```python
from build123d import *

# Parameters (mm, degrees)
SKETCH1_R           = 2.5
BOSS_EXTRUDE1_DEPTH = 6
CUT_EXTRUDE2_DEPTH  = 41.954878106


with BuildPart() as part:
    # Sketch1 → Boss-Extrude1 (new body)
    with BuildSketch(Plane.XY):
        with BuildLine():
            Line((3, 37.066220694), (3, 28.566220694))
            ThreePointArc((3, 28.566220694), (0, 25.566220694), (-3, 28.566220694))
            Line((-3, 28.566220694), (-3, 37.066220694))
            ThreePointArc((-3, 37.066220694), (0, 40.066220694), (3, 37.066220694))
        make_face()
        with Locations((0, 37.066220694)):
            Circle(SKETCH1_R, mode=Mode.SUBTRACT)
        with Locations((0, 28.566220694)):
            Circle(SKETCH1_R, mode=Mode.SUBTRACT)
    extrude(amount=BOSS_EXTRUDE1_DEPTH)

    # Sketch2 → Cut-Extrude2 (cut, through all)
    with BuildSketch(Plane.ZY.offset(3)):
        Polygon((2, 37.066220694), (2, 41.792397486), (4, 41.792397486), (4, 37.066220694), (4, 32.376323295), (2, 32.376323295), align=None)
    extrude(amount=-CUT_EXTRUDE2_DEPTH, mode=Mode.SUBTRACT)


solid = part.part
```
Geometry check sheet. Reference: the model listing, model coordinates, mm. A direction names the side the tool comes from. Round coordinates to 2 decimals unless told otherwise and drop trailing zeros. Loops run counter-clockwise (first coordinate to the right, second up) from the corner with the lowest first, then second, coordinate; pieces in that order, holes last. Notation, with made-up numbers: (36, 14.25) -> (72, 14.25) arc R17 cw to (72, 39.25) -> close; hole circle Ø5 at (57, 44). An arc over 180 degrees is marked (long way). Use a Markdown table: item, result.
(1) Mould release check, pull along Y, two halves, no side actions. Record for faces 1 (the cylindrical face through (0.066, 25.567, 2.958)), 2 (the flat face through (-1.4, 34.6, 2)), 3 (the cylindrical face through (-0.325, 31.045, 2.958)), 4 (the cylindrical face through (1.3, 39.2, 1)): released by +Y, released by -Y, zero draft, split by the parting line, or undercut.
Calculated:
| item | result |
|---|---|
| face 1 | released by -Y |
| face 2 | zero draft |
| face 3 | undercut |
| face 4 | undercut |
(2) Sectioned sample at A-A (x = 0). Enter the section's corners in (y, z), then the cut area to 3 significant figures.
Calculated:
| item | result |
|---|---|
| outline | (25.57, 0) -> (26.07, 0) -> (26.07, 6) -> (25.57, 6) -> close; (31.07, 0) -> (34.57, 0) -> (34.57, 2) -> (32.38, 2) -> (32.38, 4) -> (34.57, 4) -> (34.57, 6) -> (31.07, 6) -> close; (39.57, 0) -> (40.07, 0) -> (40.07, 2) -> (39.57, 2) -> close; (39.57, 4) -> (40.07, 4) -> (40.07, 6) -> (39.57, 6) -> close |
| area | 21.6 mm² |
(3) Sectioned sample at C-C (y = 36.25). Enter the section's corners in (x, z), then the cut area to 3 significant figures.
Calculated:
| item | result |
|---|---|
| outline | (-3, 0) -> (-2.36, 0) -> (-2.36, 2) -> (-3, 2) -> close; (-3, 4) -> (-2.36, 4) -> (-2.36, 6) -> (-3, 6) -> close; (2.36, 0) -> (3, 0) -> (3, 2) -> (2.36, 2) -> close; (2.36, 4) -> (3, 4) -> (3, 6) -> (2.36, 6) -> close |
| area | 5.10 mm² |
(4) Go/stop test with flat-tipped pins: P1, Ø1.5, axis at x = 1, z = 4.5, coming from the -Y side; P2, Ø3, axis at y = 37.5, z = 1, coming from the -X side; P3, Ø1, axis at x = -0.5, z = 3, coming from the +Y side. Record where each tip stops, or that it passes through.
Calculated:
| item | result |
|---|---|
| P1 | y = 25.58 |
| P2 | x = -3 |
| P3 | y = 32.38 |
(5) Sectioned sample at B-B (z = 4.65). Enter the section's corners in (x, y), then the cut area to 3 significant figures.
Calculated:
| item | result |
|---|---|
| outline | (-3, 28.57) arc R3 ccw to (3, 28.57) -> (3, 37.07) arc R3 ccw to (-3, 37.07) -> close; hole circle Ø5 at (0, 28.57); hole circle Ø5 at (0, 37.07) |
| area | 40.0 mm² |
(6) Scan lines: probe 1 along Y at (x, z) = (0, 0.55); probe 2 along Y at (x, z) = (0, 3.2); probe 3 along Z at (x, y) = (2.2, 33). Record each from-to range of solid material in increasing order.
Calculated:
| item | result |
|---|---|
| probe 1 | 25.57 to 26.07, 31.07 to 34.57, 39.57 to 40.07 |
| probe 2 | 25.57 to 26.07, 31.07 to 32.38 |
| probe 3 | 0 to 2, 4 to 6 |
(7) Sectioned sample at D-D (z = 2.85). Enter the section's corners in (x, y).
Calculated:
| item | result |
|---|---|
| outline | (-3, 28.57) arc R3 ccw to (3, 28.57) -> (3, 32.38) -> (-3, 32.38) -> close; hole circle Ø5 at (0, 28.57) |
(8) Set-up check for faces 5 (the flat face through (0, 34, 4)), 6 (the cylindrical face through (1.3, 39.2, 5)): record each of +Z, -Z, +X, -X, +Y, -Y from which the full face is reachable in a straight line by a thin tool's end or side.
Calculated:
| item | result |
|---|---|
| face 5 | +X, -X, +Y |
| face 6 | +Z, -Z |
